Source: CAD feature listing. Evaluate the final solid. Frame: model axes, mm. Give positions to 0.01 mm unless a question says otherwise; leave off trailing zeros. Write each loop counter-clockwise with the first axis right and the second up, starting at its lowest first coordinate (ties: lowest second). Pieces come first, ordered by that corner, then holes. Notation, with made-up numbers: (50.5, 54) -> (63.5, 54) arc R31 ccw to (63.5, 78) -> close; hole circle Ø11 at (31, 38). An arc over 180 degrees is marked (long way). Answer as a JSON object with one key per item and string values. Group by question number.
Item 1: Section query B-B on x = 41.5. Return the cut outline in (y, z).
Item 2: Section query A-A on z = 41.5. Return the cut outline in (x, y), plus the area to 3 significant figures.
Item 3: Ray query, probe 1 along Z at (x, y) = (-41.5, -7.25); probe 2 along Z at (x, y) = (-37.5, -4.75); probe 3 along X at (y, z) = (-14.5, -1). Return the intervals inside material, ascending. Write a range as from..to.
Item 4: Section query C-C on y = -7.5. Return the cut outline in (x, z).
Item 5: Section query D-D on x = 4.5. Return the cut outline in (y, z), plus the area to 3 significant figures.
from build123d import *

# Parameters (mm, degrees)
F0_W     = 120
F0_H     = 218
F0_R     = 6.25
F0_R_2   = 17.5
F1_DEPTH = 15
F2_SIZE2 = 5
F2_SIZE  = 5


with BuildPart() as f1:
    # F0 (on Front) → F1 (new body)
    with BuildSketch(Plane.XZ):
        with Locations((0, 10)):
            Rectangle(F0_W, F0_H)
        with Locations((-41.5, -41.5)):
            Circle(F0_R, mode=Mode.SUBTRACT)
        with Locations((-32.5, 0)):
            Circle(F0_R, mode=Mode.SUBTRACT)
        Circle(F0_R_2, mode=Mode.SUBTRACT)
        with Locations((41.5, -41.5)):
            Circle(F0_R, mode=Mode.SUBTRACT)
        with Locations((32.5, 0)):
            Circle(F0_R, mode=Mode.SUBTRACT)
        with Locations((-41.5, 41.5)):
            Circle(F0_R, mode=Mode.SUBTRACT)
        with Locations((41.5, 41.5)):
            Circle(F0_R, mode=Mode.SUBTRACT)
    extrude(amount=F1_DEPTH)

    # F2
    f2_edges = [f1.edges().sort_by_distance(p)[0] for p in [
        (-47.75, -15, 41.5),
        (35.25, -15, 41.5),
        (-47.75, -15, -41.5),
        (35.25, -15, -41.5),
        (60, -15, 10),
    ]]
    chamfer(f2_edges, length=F2_SIZE, length2=F2_SIZE2)


solid = f1.part
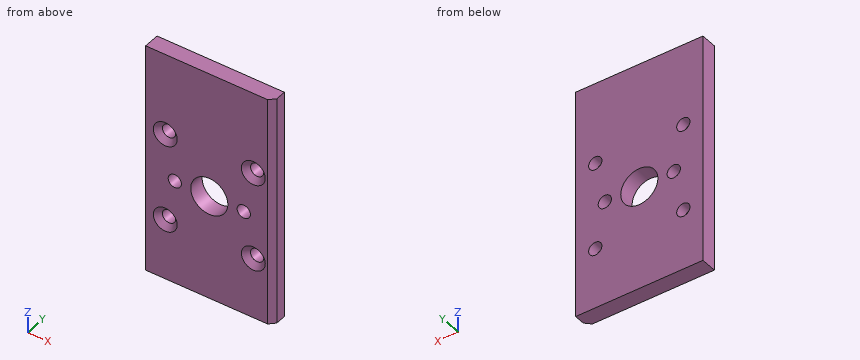
Worked answers:
{
 "1": {"outline": "(-15, -99) -> (0, -99) -> (0, -47.75) -> (-10, -47.75) -> (-15, -52.75) -> close; (-15, -30.25) -> (-10, -35.25) -> (0, -35.25) -> (0, 35.25) -> (-10, 35.25) -> (-15, 30.25) -> close; (-15, 52.75) -> (-10, 47.75) -> (0, 47.75) -> (0, 119) -> (-15, 119) -> close"},
 "2": {"outline": "(-60, -15) -> (-52.75, -15) -> (-47.75, -10) -> (-47.75, 0) -> (-60, 0) -> close; (-35.25, -10) -> (-30.25, -15) -> (30.25, -15) -> (35.25, -10) -> (35.25, 0) -> (-35.25, 0) -> close; (47.75, -10) -> (52.75, -15) -> (55, -15) -> (60, -10) -> (60, 0) -> (47.75, 0) -> close", "area": "1,360 mm^2"},
 "3": {"probe 1": "-99..-47.75, -35.25..35.25, 47.75..119", "probe 2": "-99..-46.3, -36.7..-3.75, 3.75..36.7, 46.3..119", "probe 3": "-60..-38.67, -26.33..-17.47, 17.47..26.33, 38.67..55.5"},
 "4": {"outline": "(-60, -99) -> (60, -99) -> (60, 119) -> (-60, 119) -> close; hole circle Ø12.5 at (-41.5, -41.5); hole circle Ø12.5 at (-41.5, 41.5); hole circle Ø12.5 at (-32.5, 0); hole circle Ø35 at (0, 0); hole circle Ø12.5 at (32.5, 0); hole circle Ø12.5 at (41.5, -41.5); hole circle Ø12.5 at (41.5, 41.5)"},
 "5": {"outline": "(-15, -99) -> (0, -99) -> (0, -16.91) -> (-15, -16.91) -> close; (-15, 16.91) -> (0, 16.91) -> (0, 119) -> (-15, 119) -> close", "area": "2,760 mm^2"}
}
